Verification items for the finished model (mm, model axes). A direction names the side the tool comes from. Round coordinates to 2 decimals unless told otherwise and drop trailing zeros. Order: outer loops, then holes, each group sorted by start corner. A loop starts at its lowest first (then second) coordinate and runs counter-clockwise, first axis right, second up.
```python
from build123d import *

# Parameters (mm, degrees)
SKETCH1_W                           = 34
SKETCH1_H                           = 40
SKETCH1_R                           = 8
SKETCH1_R_2                         = 2
BOSS_EXTRUDE1_DEPTH                 = 10
M4X0_7_TAPPED_HOLE1_D               = 3.3
M4X0_7_TAPPED_HOLE1_DEPTH           = 15
M4X0_7_TAPPED_HOLE1_TIP             = 0.991420021
M4X0_7_TAPPED_HOLE1_ON_FACE_2_D     = 3.3
M4X0_7_TAPPED_HOLE1_ON_FACE_2_DEPTH = 15
M4X0_7_TAPPED_HOLE1_ON_FACE_2_TIP   = 0.991420021


with BuildPart() as part:
    # Sketch1 → Boss-Extrude1 (new body)
    with BuildSketch(Plane(origin=(0, 0, 0), x_dir=(1, 0, 0), z_dir=(0, 1, 0))):
        Rectangle(SKETCH1_W, SKETCH1_H)
        with Locations(Location((0, 0, 0), (0, 0, 270))):
            Circle(SKETCH1_R, mode=Mode.SUBTRACT)
        with Locations(Location((0, 13.75, 0), (0, 0, 270))):
            Circle(SKETCH1_R_2, mode=Mode.SUBTRACT)
        with Locations(Location((0, -13.75, 0), (0, 0, 270))):
            Circle(SKETCH1_R_2, mode=Mode.SUBTRACT)
        with Locations(Location((-12.5, 0, 0), (0, 0, 270))):
            Circle(SKETCH1_R_2, mode=Mode.SUBTRACT)
        with Locations(Location((12.5, 0, 0), (0, 0, 270))):
            Circle(SKETCH1_R_2, mode=Mode.SUBTRACT)
    extrude(amount=BOSS_EXTRUDE1_DEPTH)

    # M4x0.7 Tapped Hole1
    with Locations(Plane(origin=(9.5, 5, -20), x_dir=(-1, 0, 0), z_dir=(0, 0, -1))):
        with Locations((0, 0), (19, 0)):
            Hole(M4X0_7_TAPPED_HOLE1_D / 2, depth=M4X0_7_TAPPED_HOLE1_DEPTH)
            with Locations((0, 0, -(M4X0_7_TAPPED_HOLE1_DEPTH + M4X0_7_TAPPED_HOLE1_TIP / 2))):  # 118° drill point
                Cone(0, M4X0_7_TAPPED_HOLE1_D / 2, M4X0_7_TAPPED_HOLE1_TIP, mode=Mode.SUBTRACT)

    # M4x0.7 Tapped Hole1 on face 2
    with Locations(Plane(origin=(-9.5, 5, 20), x_dir=(1, 0, 0), z_dir=(0, 0, 1))):
        with Locations((0, 0), (19, 0)):
            Hole(M4X0_7_TAPPED_HOLE1_ON_FACE_2_D / 2, depth=M4X0_7_TAPPED_HOLE1_ON_FACE_2_DEPTH)
            with Locations((0, 0, -(M4X0_7_TAPPED_HOLE1_ON_FACE_2_DEPTH + M4X0_7_TAPPED_HOLE1_ON_FACE_2_TIP / 2))):  # 118° drill point
                Cone(0, M4X0_7_TAPPED_HOLE1_ON_FACE_2_D / 2, M4X0_7_TAPPED_HOLE1_ON_FACE_2_TIP, mode=Mode.SUBTRACT)


solid = part.part
```
1) Sectioned sample at C-C on z = 0. Record the cut outline in (x, y), then the cut area to 3 significant figures.
2) Scan lines: probe 1 along X at (y, z) = (6.5, 0); probe 2 along X at (y, z) = (3.5, -9.5); probe 3 along X at (y, z) = (5, 16.5). Record each from-to range of solid material in increasing order.
3) Sectioned sample at A-A on z = -13.75. Record the cut outline in (x, y), then the cut area to 3 significant figures.
4) Sectioned sample at D-D on x = -12.5. Record the cut outline in (y, z), then the cut area to 3 significant figures.
5) Draft check along Y on faces 1 (the flat face through (7, 10, -5)), 2 (the flat face through (0, 5, 20)), 3 (the cylindrical face through (-9.1, 3.4, 12.4)). Enter one of: released by +Y, released by -Y, zero draft, split by the parting line, or undercut.
6) Sectioned sample at B-B on x = 0. Record the cut outline in (y, z).
7) Tool access check on faces 4 (the cylindrical face through (-9.9, 3.4, -12.4)), 5 (the cylindrical face through (9.9, 3.4, 12.4)), 6 (the cylindrical face through (-10.517, 4.93, -0.26)). Record the directions out of +Z, -Z, +X, -X, +Y, -Y that give a thin tool (end or side, any length) a straight path to the whole face; none if there is none.
8) Go/stop test with flat-tipped pins: pin 1 Ø3 at (x, y) = (9.5, 5) entering from +Z; pin 2 Ø2.5 at (x, z) = (0, 13.75) entering from +Y (3 decimals). Record where each tip stops, or that it passes through.
Returned:
1. outline: (-17, 0) - (-14.5, 0) - (-14.5, 10) - (-17, 10) - close; (-10.5, 0) - (-8, 0) - (-8, 10) - (-10.5, 10) - close; (8, 0) - (10.5, 0) - (10.5, 10) - (8, 10) - close; (14.5, 0) - (17, 0) - (17, 10) - (14.5, 10) - close
1. area: 100 mm2
2. probe 1: x = -17 to -14.5, -10.5 to -8, 8 to 10.5, 14.5 to 17
2. probe 2: x = -17 to -10.19, -8.81 to 8.81, 10.19 to 17
2. probe 3: x = -17 to -11.15, -7.85 to 7.85, 11.15 to 17
3. outline: (-17, 0) - (-2, 0) - (-2, 10) - (-17, 10) - close; (2, 0) - (17, 0) - (17, 10) - (2, 10) - close; hole circle Ø3.3 at (-9.5, 5); hole circle Ø3.3 at (9.5, 5)
3. area: 283 mm2
4. outline: (0, -20) - (10, -20) - (10, -2) - (0, -2) - close; (0, 2) - (10, 2) - (10, 20) - (0, 20) - close
4. area: 360 mm2
5. face 1: released by +Y
5. face 2: zero draft
5. face 3: undercut
6. outline: (0, -20) - (10, -20) - (10, -15.75) - (0, -15.75) - close; (0, -11.75) - (10, -11.75) - (10, -8) - (0, -8) - close; (0, 8) - (10, 8) - (10, 11.75) - (0, 11.75) - close; (0, 15.75) - (10, 15.75) - (10, 20) - (0, 20) - close
7. face 4: -Z
7. face 5: +Z
7. face 6: +Y, -Y
8. pin 1: stops at z = 4.91
8. pin 2: passes through
